Answer from the drawing. Dimensions are ordinates in mm from the lowest x, y and z of the part. A direction names the side the tool comes from. Give positions to 0.01 mm unless a question says otherwise; leave off trailing zeros. Order: outer loops, then holes, each group sorted by start corner. A loop starts at its lowest first (then second) coordinate and runs counter-clockwise, first axis right, second up. Notation, with made-up numbers: (28.25, 55.5) -> (54.25, 55.5) arc R9 ccw to (54.25, 66.5) -> close; hole circle Ø11 at (44.5, 0.5). An arc over 180 degrees is marked (long way). Answer as CSV lines item,"result". Start each with the question number.
1) Find section D-D (y = 16.5). Determine the outline of the cut face in (x, z), and give its area (3 significant figures).
2) Find section B-B (x = 18). Determine the outline of the cut face in (y, z).
3) Find section C-C (y = 7.5). Determine the outline of the cut face in (x, z).
4) Find section A-A (z = 10). Determine the outline of the cut face in (x, y).
5) The mould has two halves that part along Z. Classify the marked faces 1, 2, 3 and 4: +Z half, -Z half, draft (parallel to the pull), parting line (faces both ways), or undercut.
6) For the marked faces 5, 6 and 7, determine the directions among +Z, -Z, +X, -X, +Y, -Y from which every point of the face is accessible in a straight line to the end or side of a thin tool.
7) Flat-ended cylindrical pins translate along their axes: pin 1 Ø1.2 at (y, z) = (23, 19) entering from +X; pin 2 Ø2 at (x, z) = (25, 1) entering from +Y; pin 3 Ø2 at (y, z) = (21, 5.5) entering from +X. Find the tip coordinate at first contact, or state that the pin passes through.
8) Straight lines are drawn through the part: L1, parallel to Z at x = 21.25, y = 4.5; L2, parallel to Y at x = 1.2, z = 10; L3, parallel to Y at x = 12.5, z = 9.75. For each, find the intervals that lie inside material, in ascending order. Write a range as from..to.
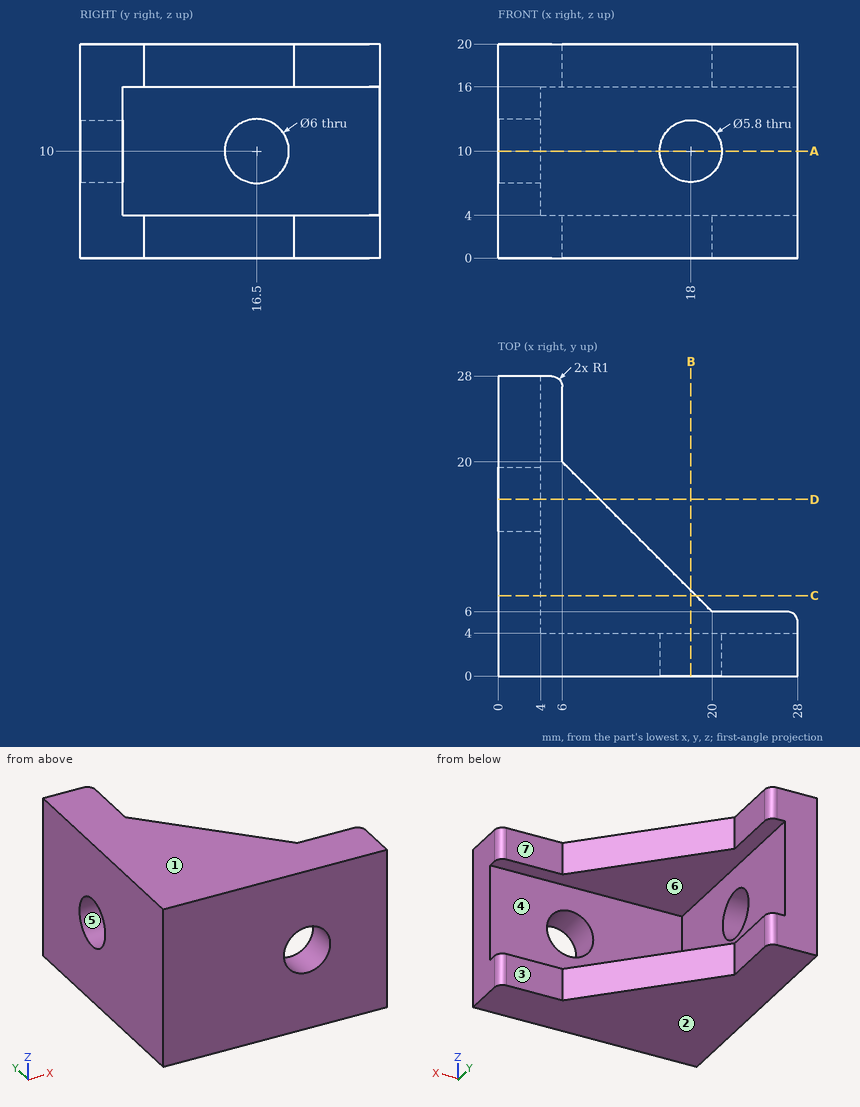
Findings below:
1,outline,"(0, 0) -> (9.5, 0) -> (9.5, 4) -> (4, 4) -> (4, 7) -> (0, 7) -> close; (0, 13) -> (4, 13) -> (4, 16) -> (9.5, 16) -> (9.5, 20) -> (0, 20) -> close"
1,area,"100 mm²"
2,outline,"(0, 0) -> (8, 0) -> (8, 4) -> (4, 4) -> (4, 7.1) -> (0, 7.1) -> close; (0, 12.9) -> (4, 12.9) -> (4, 16) -> (8, 16) -> (8, 20) -> (0, 20) -> close"
3,outline,"(0, 0) -> (18.5, 0) -> (18.5, 4) -> (4, 4) -> (4, 16) -> (18.5, 16) -> (18.5, 20) -> (0, 20) -> close"
4,outline,"(0, 0) -> (15.1, 0) -> (15.1, 4) -> (4, 4) -> (4, 13.5) -> (0, 13.5) -> close; (0, 19.5) -> (4, 19.5) -> (4, 28) -> (0, 28) -> close; (20.9, 0) -> (28, 0) -> (28, 4) -> (20.9, 4) -> close"
5,face 1,"+Z half"
5,face 2,"-Z half"
5,face 3,"draft"
5,face 4,"undercut"
6,face 5,"+X, -X"
6,face 6,"+X, +Y"
6,face 7,"+Z, -Z, +X, +Y"
7,pin 1,"x = 6"
7,pin 2,"y = 6"
7,pin 3,"x = 4"
8,L1,"0..4, 16..20"
8,L2,"0..13.5, 19.5..28"
8,L3,"0..4"
